from build123d import *

# Parameters (mm, degrees)
SKETCH1_R           = 15
BOSS_EXTRUDE1_DEPTH = 1.5875


with BuildPart() as part:
    # Sketch1 → Boss-Extrude1 (new body)
    with BuildSketch(Plane(origin=(0, 0, 0), x_dir=(1, 0, 0), z_dir=(0, 1, 0))):
        Polygon((0, 27.5), (0, 0), (30, 0), (30, 6.35), (50, 6.35), (50, 0), (70, 0), (70, 6.35), (90, 6.35), (90, 0), (110, 0), (110, 6.35), (130, 6.35), (130, 0), (150, 0), (150, 6.35), (170, 6.35), (170, 0), (200, 0), (200, 27.5), (193.65, 27.5), (193.65, 47.5), (200, 47.5), (200, 75), (170, 75), (170, 68.65), (150, 68.65), (150, 75), (130, 75), (130, 68.65), (110, 68.65), (110, 75), (90, 75), (90, 68.65), (70, 68.65), (70, 75), (50, 75), (50, 68.65), (30, 68.65), (30, 75), (0, 75), (0, 47.5), (6.35, 47.5), (6.35, 27.5), align=None)
        with Locations((100, 37.5)):
            Circle(SKETCH1_R, mode=Mode.SUBTRACT)
    extrude(amount=BOSS_EXTRUDE1_DEPTH)


solid = part.part
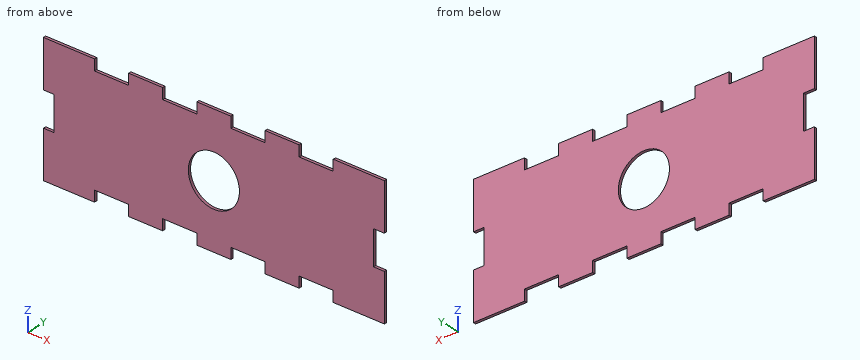
Design review of the part built by this model. Coordinates are the model's own, in mm. Give positions to 0.01 mm unless a question says otherwise; leave off trailing zeros. Loops run counter-clockwise (first coordinate to the right, second up) from the corner with the lowest first, then second, coordinate; pieces in that order, holes last. Notation, with made-up numbers: M 35.25,16 L 45.25,16 A24 cw 45.25,43 Z; hole C 78,78 d8. An arc over 180 degrees is marked long. One line per question, with ' | ' between items. Start each with the question number.
1. Add section A-A (x = 100). Write out the cut boundary in (y, z), plus the area to 3 significant figures.
2. Insertion check: P1, Ø0.5, axis at y = 0.5, z = -70.5, coming from the -X side; P2, Ø0.5, axis at x = 84, y = 1, coming from the +Z side. Each pin has a flat end and moves straight along its axis. Give the tip position at first contact, or say it passes through.
3. To check wall thickness, follow L1, parallel to X at y = 0.7, z = -37.5; L2, parallel to Z at x = 100, y = 0.75; L3, parallel to X at y = 0.6, z = -43. State the ranges of each line that lie inside material, in increasing order.
4. Add section B-B (z = -37.5). Write out the cut boundary in (x, y).
Worked out:
1) outline: M 0,-75 L 1.59,-75 L 1.59,-52.5 L 0,-52.5 Z; M 0,-22.5 L 1.59,-22.5 L 1.59,0 L 0,0 Z | area: 71.4 mm²
2) P1: stops at x = 0 | P2: stops at z = -6.35
3) L1: x = 6.35 to 85, 115 to 193.65 | L2: z = -75 to -52.5, -22.5 to 0 | L3: x = 6.35 to 86.04, 113.96 to 193.65
4) outline: M 6.35,0 L 85,0 L 85,1.59 L 6.35,1.59 Z; M 115,0 L 193.65,0 L 193.65,1.59 L 115,1.59 Z
